The model under review builds one solid part; all positions refer to its coordinate system, in mm. Round coordinates to 2 decimals unless told otherwise and drop trailing zeros. Loops run counter-clockwise (first coordinate to the right, second up) from the corner with the lowest first, then second, coordinate; pieces in that order, holes last. Notation, with made-up numbers: M -36,-34 L -32,-34 A29 ccw -32,-7 Z; hole C 27.25,0 d6. An arc over 180 degrees is marked long. Return JSON: item names as keys, results as strings. Group by question number.
Q1. Consider section A-A (x = 0). State the section outline as (y, z) points.
Q2. Consider section D-D (z = -12). State the section outline as (x, y) points.
Q3. Consider section C-C (x = -1.6). State the section outline as (y, z) points, and give its area (3 significant figures).
Q4. Consider section B-B (y = 0.15). State the section outline as (x, z) points, and give its area (3 significant figures).
Q5. To check wall thickness, follow line 1 along X through (y, z) = (0, 1.5); line 2 along Z through (x, y) = (-2.4, 0); line 3 along X through (y, z) = (-0.1, -6.75). State the ranges of each line that lie inside material, in increasing order.
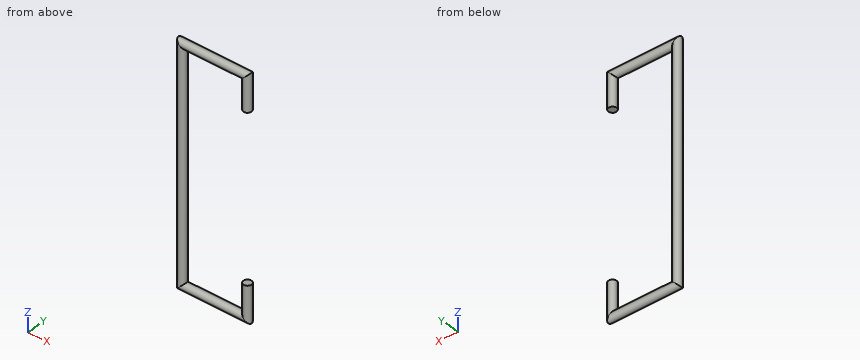
Autodesk Inventor part; units mm, degrees
ref_plane "YZ Plane" through (0, 0, 0) normal (1, 0, 0) x (0, 1, 0)
ref_plane "XZ Plane" through (0, 0, 0) normal (0, 1, 0) x (-1, 0, 0)
ref_plane "XY Plane" through (0, 0, 0) normal (0, 0, 1) x (1, 0, 0)
sketch "Skizze1" plane through (0, 0, 0) normal (0, 0, 1) x (1, 0, 0)
  circle A0 centre (0, 0) radius 0.25
  dimension "d0" = 0.5
sketch "Skizze2" plane through (0, 0, 0) normal (0, 1, 0) x (-1, 0, 0)
  line L0 (0, 0) -> (0, 2)
  line L1 (0, 2) -> (4, 2)
  line L2 (4, 2) -> (4, -12)
  line L3 (4, -12) -> (0, -12)
  line L4 (0, -12) -> (0, -10)
  dimension "d1" = 2
  dimension "d2" = 4
  dimension "d3" = 14
  dimension "d4" = 2
sweep "Sweeping1" add profiles "Skizze1" path "Skizze2"
properties part number "Transition_3_Init"
Values:
{
 "1": {"outline": "M -0.25,-12 A0.25 ccw 0.25,-12 L 0.25,-10 L -0.25,-10 Z; M -0.25,0 L 0.25,0 L 0.25,2 A0.25 ccw -0.25,2 Z"},
 "2": {"outline": "M -4,-0.25 L 0,-0.25 A0.25 ccw 0,0.25 L -4,0.25 A0.25 ccw Z"},
 "3": {"outline": "C 0,-12 d0.5; C 0,2 d0.5", "area": "0.393 mm2"},
 "4": {"outline": "M -4.2,-12.2 L 0.2,-12.2 L 0.2,-10 L -0.2,-10 L -0.2,-11.8 L -3.8,-11.8 L -3.8,1.8 L -0.2,1.8 L -0.2,0 L 0.2,0 L 0.2,2.2 L -4.2,2.2 Z", "area": "10.4 mm2"},
 "5": {"line 1": "x = -4.25 to -3.75, -0.25 to 0.25", "line 2": "z = -12.25 to -11.75, 1.75 to 2.25", "line 3": "x = -4.23 to -3.77"}
}
